Could you check a few things on this model? Use its own coordinates, in mm. Give positions to 0.01 mm unless a question says otherwise; leave off trailing zeros. Loops run counter-clockwise (first coordinate to the right, second up) from the corner with the lowest first, then second, coordinate; pieces in that order, holes last. Notation, with made-up numbers: (56.25, 32) - (77.25, 32) arc R18 cw to (77.25, 49) - close; hole circle Ø7 at (-16, -20.5). An arc over 180 degrees is marked (long way). Write each question's results on one line, items separated by ' | '. Start each with the question number.
(1) I need wall thicknesses on line 1 (X direction, y = -5, z = -1); line 2 (Y direction, x = 12, z = -4.5) (3 decimals); line 3 (X direction, y = -4.75, z = -3.5). Which ranges of each line are inside material? Lowest first, please.
(2) Suppose I cut it at A-A (x = 8.5). Please give me the cut outline in (y, z) (3 decimals).
(3) Suppose I cut it at D-D (z = -3.5). Please give me the cut outline in (x, y) (3 decimals).
(4) If we mould it in two halves opening along Y, with no side actions, what happens to faces 1 (the face through (-9.836, -5.725, -3.131)), 2 (the face through (0, 0, -6.35)), 3 (the face through (0.22, 8.03, -1.68))? For each: released by +Y, released by -Y, zero draft, split by the parting line, or undercut.
(5) Suppose I cut it at C-C (z = -1.25). Please give me the cut outline in (x, y) (3 decimals).
(6) Suppose I cut it at B-B (y = 4.25). Please give me the cut outline in (x, z), and give its area (3 significant figures).
from build123d import *

# Parameters (mm, degrees)
BOSS_EXTRUDE1_DEPTH       = 16
F_6_32_TAPPED_HOLE1_D     = 2.7051
F_6_32_TAPPED_HOLE1_DEPTH = 9.398
F_6_32_TAPPED_HOLE1_TIP   = 0.81269403
FILLET1_R                 = 0.75
F_6_CLEARANCE_HOLE2_D     = 3.6576


with BuildPart() as part:
    # Sketch1 → Boss-Extrude1 (new, symmetric)
    with BuildSketch(Plane(origin=(0, 0, 0), x_dir=(0, 0, -1), z_dir=(1, 0, 0))):
        Polygon((0, 6.35), (3.175, 9.525), (6.35, 9.525), (6.35, -9.525), (0, -9.525), align=None)
    extrude(amount=BOSS_EXTRUDE1_DEPTH, both=True)

    # #6-32 Tapped Hole1
    with Locations(Plane(origin=(0, 0, -6.35), x_dir=(-1, 0, 0), z_dir=(0, 0, -1))):
        with Locations((11.525, 5.025), (-11.525, 5.025)):
            Hole(F_6_32_TAPPED_HOLE1_D / 2, depth=F_6_32_TAPPED_HOLE1_DEPTH)
            with Locations((0, 0, -(F_6_32_TAPPED_HOLE1_DEPTH + F_6_32_TAPPED_HOLE1_TIP / 2))):  # 118° drill point
                Cone(0, F_6_32_TAPPED_HOLE1_D / 2, F_6_32_TAPPED_HOLE1_TIP, mode=Mode.SUBTRACT)

    # Fillet1
    # the kernel refuses this fillet: 0.75 mm, written as the material it takes off along each edge
    with BuildSketch(Plane(origin=(-16.776650429, 6.35, 0), x_dir=(0, 0.707106781186552, -0.7071067811865431), z_dir=(1, 0, 0)), Plane(origin=(11.019949465, 6.35, 0), x_dir=(0, 0.707106781186552, -0.7071067811865431), z_dir=(1, 0, 0))) as fillet1_piece_1:
        with BuildLine():
            CenterArc((FILLET1_R * 0.414213562373, -FILLET1_R), FILLET1_R, 90, 45)
            Line((-FILLET1_R * 0.292893218813, -FILLET1_R * 0.292893218813), (0, 0))
            Line((0, 0), (FILLET1_R * 0.414213562373, 0))
        make_face()
    extrude(amount=5.756700965, mode=Mode.SUBTRACT)
    with BuildSketch(Plane(origin=(-12.030050535, 6.35, 0), x_dir=(0, 0.707106781186552, -0.7071067811865431), z_dir=(1, 0, 0))) as fillet1_piece_2:
        with BuildLine():
            CenterArc((FILLET1_R * 0.414213562373, -FILLET1_R), FILLET1_R, 90, 45)
            Line((-FILLET1_R * 0.292893218813, -FILLET1_R * 0.292893218813), (0, 0))
            Line((0, 0), (FILLET1_R * 0.414213562373, 0))
        make_face()
    extrude(amount=24.060101071, mode=Mode.SUBTRACT)
    with BuildSketch(Plane(origin=(-17.875, -9.525, 0), x_dir=(0, 1, 0), z_dir=(1, 0, 0))) as fillet1_piece_3:
        with BuildLine():
            CenterArc((FILLET1_R, -FILLET1_R), FILLET1_R, 90, 90)
            Line((0, -FILLET1_R), (0, 0))
            Line((0, 0), (FILLET1_R, 0))
        make_face()
    extrude(amount=35.75, mode=Mode.SUBTRACT)

    # #6 Clearance Hole2 (through all)
    with Locations(Plane(origin=(0, 0, -6.35), x_dir=(-1, 0, 0), z_dir=(0, 0, -1))):
        with Locations((-11.525, -5.025), (11.525, -5.025)):
            Hole(F_6_CLEARANCE_HOLE2_D / 2)


solid = part.part
Output values:
1) line 1: -16 to -13.35, -9.7 to 9.7, 13.35 to 16 | line 2: -9.525 to -6.791, -3.259 to 3.759, 6.291 to 9.525 | line 3: -16 to -13.33, -9.72 to 9.72, 13.33 to 16
2) outline: (-9.525, -6.35) - (9.525, -6.35) - (9.525, -3.175) - (6.57, -0.22) arc R0.75 ccw to (6.039, 0) - (-8.775, 0) arc R0.75 ccw to (-9.525, -0.75) - close
3) outline: (-16, -9.525) - (16, -9.525) - (16, 9.525) - (-16, 9.525) - close; hole circle Ø3.658 at (-11.525, -5.025); hole circle Ø2.705 at (-11.525, 5.025); hole circle Ø3.658 at (11.525, -5.025); hole circle Ø2.705 at (11.525, 5.025)
4) face 1: undercut | face 2: zero draft | face 3: released by +Y
5) outline: (-16, -9.525) - (16, -9.525) - (16, 7.6) - (-16, 7.6) - close; hole circle Ø3.658 at (-11.525, -5.025); hole circle Ø2.705 at (-11.525, 5.025); hole circle Ø3.658 at (11.525, -5.025); hole circle Ø2.705 at (11.525, 5.025)
6) outline: (-16, -6.35) - (-12.63, -6.35) - (-12.63, 0) - (-16, 0) - close; (-10.42, -6.35) - (10.42, -6.35) - (10.42, 0) - (-10.42, 0) - close; (12.63, -6.35) - (16, -6.35) - (16, 0) - (12.63, 0) - close | area: 175 mm2
